from build123d import *

# Parameters (mm, degrees)
SKETCH2_R           = 11
BOSS_EXTRUDE1_DEPTH = 6
SKETCH3_W           = 3.45
SKETCH3_H           = 3.45
CUT_EXTRUDE1_DEPTH  = 18.841034143
SKETCH4_R           = 13
BOSS_EXTRUDE2_DEPTH = 1.5
SKETCH5_W           = 3.45
SKETCH5_H           = 3.45
CUT_EXTRUDE2_DEPTH  = 22.625712586
SKETCH6_R           = 2.6
CUT_EXTRUDE3_DEPTH  = 22.625712586


with BuildPart() as part:
    # Sketch2 → Boss-Extrude1 (new body)
    with BuildSketch(Plane(origin=(-0.006046198, 2.843115255, 0.024063532), x_dir=(0.9999977389340391, 0.002126453123543878, 1.7997853821493017e-05), z_dir=(-0.00212652928721231, 0.9999619230641714, 0.008463468260412206))):
        with Locations(Location((-2.8797e-05, 1.599942694, 0), (0, 0, 270))):
            Circle(SKETCH2_R)
    extrude(amount=BOSS_EXTRUDE1_DEPTH)

    # Sketch3 → Cut-Extrude1 (cut, through all)
    with BuildSketch(Plane(origin=(-0.018805374, 8.842886793, 0.074844342), x_dir=(0.9999977389340391, 0.002126453123543878, 1.7997853821493024e-05), z_dir=(-0.00212652928721231, 0.9999619230641714, 0.00846346826041221))):
        with Locations((-2.8797e-05, 1.599942694)):
            Rectangle(SKETCH3_W, SKETCH3_H)
    extrude(amount=-CUT_EXTRUDE1_DEPTH, mode=Mode.SUBTRACT)

    # Sketch4 → Boss-Extrude2 (add)
    with BuildSketch(Plane(origin=(-0.018805374, 8.842886793, 0.074844342), x_dir=(0.9999977389340391, 0.002126453123543878, 1.7997853821493024e-05), z_dir=(-0.00212652928721231, 0.9999619230641714, 0.00846346826041221))):
        with Locations(Location((-2.8797e-05, 1.599942694, 0), (0, 0, 270))):
            Circle(SKETCH4_R)
    boss_extrude2 = extrude(amount=BOSS_EXTRUDE2_DEPTH)

    # Mirror1: Boss-Extrude2 across plane
    add(boss_extrude2.mirror(Plane(origin=(-0.012425786, 5.843001024, 0.049453937), x_dir=(1.79984577561216e-05, -0.008463449122581367, 0.9999641842111171), z_dir=(0.00212652928721231, -0.9999619230641714, -0.00846346826041221))))

    # Sketch5 → Cut-Extrude2 (cut, through all)
    with BuildSketch(Plane(origin=(-0.021995168, 10.342829678, 0.087539544), x_dir=(0.9999977389340391, 0.002126453123543878, 1.799785382149303e-05), z_dir=(-0.00212652928721231, 0.9999619230641714, 0.008463468260412213))):
        with Locations((-2.8797e-05, 1.599942694)):
            Rectangle(SKETCH5_W, SKETCH5_H)
    extrude(amount=-CUT_EXTRUDE2_DEPTH, mode=Mode.SUBTRACT)

    # Sketch6 → Cut-Extrude3 (cut, through all)
    with BuildSketch(Plane(origin=(-0.021995168, 10.342829678, 0.087539544), x_dir=(0.9999977389340391, 0.002126453123543878, 1.799785382149303e-05), z_dir=(-0.00212652928721231, 0.9999619230641714, 0.008463468260412213))):
        with Locations(Location((-2.8797e-05, 1.599942694, 0), (0, 0, 270))):
            Circle(SKETCH6_R)
    extrude(amount=-CUT_EXTRUDE3_DEPTH, mode=Mode.SUBTRACT)


solid = part.part
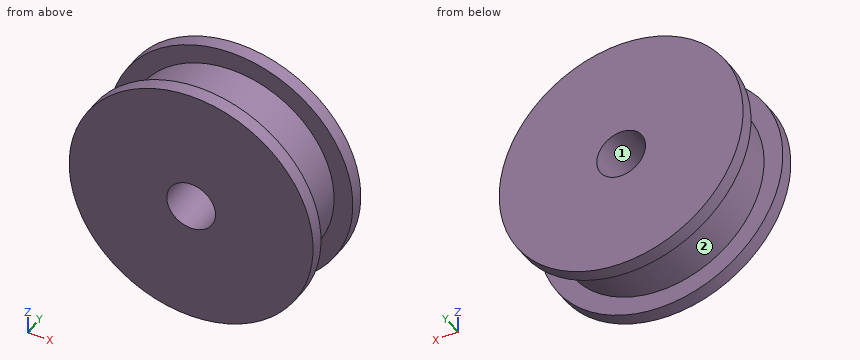
CAD build for the part. Positions are in the model's coordinates, mm. Face numbers are marked on the shaded views. Round coordinates to 2 decimals unless told otherwise and drop trailing zeros. Put each result on its own line as item: value. Start each with the question number.
1) Pull direction X, two halves, no side cores. Call the marked faces 1 and 2: pulls with the +X half, pulls with the -X half, needs draft (parallel to the pull), parting line crosses it, or undercut.
2) Pin check, flat tips, straight feed: pin 1 Ø8 at (x, z) = (-5, 5) entering from -Y; pin 2 Ø5 at (y, z) = (5.5, 7) entering from -X; pin 3 Ø2 at (x, y) = (2, 3.5) entering from +Z. Stop position of each tip, or through.
3) Drill centre lines: probe 1 along Y at (x, z) = (-11.75, -6); probe 2 along X at (y, z) = (8.75, -2.5); probe 3 along Z at (x, y) = (1, 6). Where is each one in solid material? Low to high. Write a range as [from, to].
Resolved:
1. face 1: undercut
1. face 2: parting line crosses it
2. pin 1: y = 1.26
2. pin 2: x = -9.2
2. pin 3: z = 11.35
3. probe 1: [1.37, 2.87], [8.87, 10.37]
3. probe 2: [-10.98, -2.43], [2.39, 10.94]
3. probe 3: [-12.5, -3.94], [0.85, 9.4]
